Part model, mm, in its own coordinate system. Face numbers are marked on the shaded views. A direction names the side the tool comes from. Round coordinates to 2 decimals unless told otherwise and drop trailing zeros. Loops run counter-clockwise (first coordinate to the right, second up) from the corner with the lowest first, then second, coordinate; pieces in that order, holes last. Notation, with made-up numbers: M 14.25,54 L 73.25,54 A12 ccw 73.25,68 Z; hole C -37,36 d7. An arc over 180 degrees is marked long. Put each result on its own line as item: value. Start each with the question number.
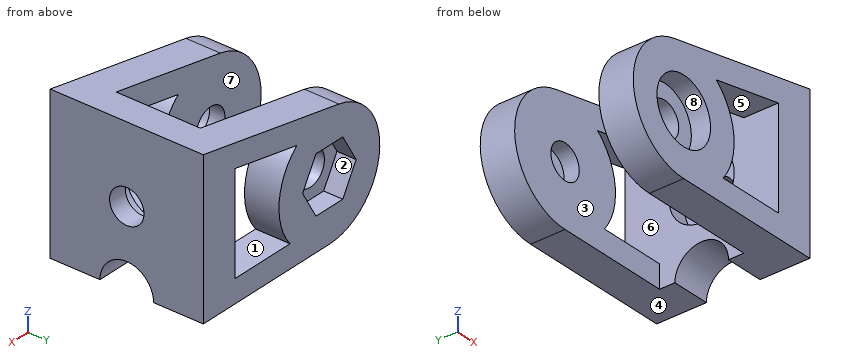
```python
from build123d import *

# Parameters (mm, degrees)
SKETCH024_R       = 2.25
PAD018_DEPTH      = 10
CYLINDER062_R     = 3.5
CYLINDER062_DEPTH = 5
BOX001_W          = 26
BOX001_H          = 11
BOX001_DEPTH      = 20
CYLINDER065_R     = 2.25
CYLINDER065_DEPTH = 5
CYLINDER066_R     = 4.25
CYLINDER066_DEPTH = 2.5
CYLINDER067_R     = 4.25
CYLINDER067_DEPTH = 2.5
POCKET008_DEPTH   = 2.5


with BuildPart() as part:
    # Sketch024 → Pad018 (new body, symmetric)
    with BuildSketch(Plane.XZ):
        with BuildLine():
            ThreePointArc((-1.513336, 7.85556), (-7.963808, -0.760107), (0, -8))
            Line((0, -8), (20, -8))
            Line((20, 12), (20, -8))
            Line((20, 12), (-1.513336, 7.85556))
        make_face()
        Circle(SKETCH024_R, mode=Mode.SUBTRACT)
        with BuildLine():
            Line((5.168757, 6.106058), (15, 8))
            Line((15, 8), (15, -5))
            Line((15, -5), (6.244998, -5))
            ThreePointArc((6.244998, -5), (7.9627, 0.771631), (5.168757, 6.106058))
        make_face(mode=Mode.SUBTRACT)
    extrude(amount=PAD018_DEPTH, both=True)

    # Cylinder062 → Cylinder062 (cut)
    with BuildSketch(Plane(origin=(15, 0, -8), x_dir=(0, 1, 0), z_dir=(1, 0, 0))):
        Circle(CYLINDER062_R)
    extrude(amount=CYLINDER062_DEPTH, mode=Mode.SUBTRACT)

    # Box001 → Box001 (cut)
    with BuildSketch(Plane(origin=(-11, -5.5, -8), x_dir=(1, 0, 0), z_dir=(0, 0, 1))):
        with Locations((13, 5.5)):
            Rectangle(BOX001_W, BOX001_H)
    extrude(amount=BOX001_DEPTH, mode=Mode.SUBTRACT)

    # Cylinder065 → Cylinder065 (cut)
    with BuildSketch(Plane(origin=(15, 0, 2), x_dir=(0, 1, 0), z_dir=(1, 0, 0))):
        Circle(CYLINDER065_R)
    extrude(amount=CYLINDER065_DEPTH, mode=Mode.SUBTRACT)

    # Cylinder066 → Cylinder066 (cut)
    with BuildSketch(Plane(origin=(15, 0, 2), x_dir=(0, 1, 0), z_dir=(1, 0, 0))):
        Circle(CYLINDER066_R)
    extrude(amount=CYLINDER066_DEPTH, mode=Mode.SUBTRACT)

    # Cylinder067 → Cylinder067 (cut)
    with BuildSketch(Plane.XZ.offset(7.5)):
        Circle(CYLINDER067_R)
    extrude(amount=CYLINDER067_DEPTH, mode=Mode.SUBTRACT)

    # Sketch040 (on Face2 of Cylinder067) → Pocket008 (cut)
    with BuildSketch(Plane(origin=(0, 10, 0), x_dir=(1, 0, 0), z_dir=(0, 1, 0))):
        Polygon((4.25, 0), (2.125, 3.680608), (-2.125, 3.680608), (-4.25, 0), (-2.125, -3.680608), (2.125, -3.680608), align=None)
    extrude(amount=-POCKET008_DEPTH, mode=Mode.SUBTRACT)


solid = part.part
```
1. Which spindle directions (+Z, -Z, +X, -X, +Y, -Y) get a long thin tool onto all of the face, cutting with end or side? Do the marked faces 5, 6, 7 and 8. Say none if no direction does.
2. Cut at A-A, the plane y = 0. Give the cut face in (x, z).
3. Cut at C-C, the plane x = -6. Give the cut face in (y, z).
4. Mould opens along Z. For the marked faces 1, 2, 3 and 4 say: released by +Z, released by -Z, zero draft, split by the parting line, or undercut.
5. Wall check: L1, parallel to X at y = -6.9, z = 0; L2, parallel to Y at x = 14.25, z = 8; L3, parallel to X at y = 1.75, z = 8.5. Give the ranges that are in metal, low to high.
6. Drop flat-ended pins along their axis: pin 1 (1.3 mm diameter, centred on x = 11, y = 6.5, fed in from +Z); pin 2 (6 mm diameter, centred on x = 0, z = 0, fed in from -Y); pin 3 (1.3 mm diameter, centred on x = 9.5, y = -7, fed in from +Z). Give the stop position or say it passes through.
7. Cut at B-B, the plane z = -1. Give the number of separate pieces and of enclosed holes in the cut face, and give its area (3 significant figures).
8. Cut at D-D, the plane z = 7. Give the cut face in (x, y), and give its area (3 significant figures).
Results list:
1. face 5: +Y, -Y
1. face 6: none
1. face 7: +Z, -Z, -X
1. face 8: -Y
2. outline: M 15,-4.5 L 20,-4.5 L 20,-0.25 L 17.5,-0.25 L 17.5,-2.25 L 15,-2.25 Z; M 15,6.25 L 17.5,6.25 L 17.5,4.25 L 20,4.25 L 20,12 L 15,11.04 Z
3. outline: M -10,-5.29 L -5.5,-5.29 L -5.5,5.29 L -10,5.29 Z; M 5.5,-5.29 L 10,-5.29 L 10,5.29 L 5.5,5.29 Z
4. face 1: undercut
4. face 2: undercut
4. face 3: zero draft
4. face 4: released by -Z
5. L1: x = -8 to -2.25, 2.25 to 8, 15 to 20
5. L2: y = -10 to -5.5, 5.5 to 10
5. L3: x = 15 to 20
6. pin 1: stops at z = 10.39
6. pin 2: stops at y = -7.5
6. pin 3: stops at z = 10.1
7. separate pieces: 5
7. enclosed holes: 0
7. area: 173 mm^2
8. outline: M -3.87,-10 L 9.81,-10 L 9.81,-5.5 L -3.87,-5.5 Z; M -3.87,5.5 L 9.81,5.5 L 9.81,10 L -3.87,10 Z; M 15,-10 L 20,-10 L 20,10 L 15,10 Z
8. area: 223 mm^2
